from build123d import *

# Parameters (mm, degrees)
UNDERSIDE_COVER_T2_DEPTH         = 2
SKETCH_2_R                       = 1.7
CLOSURE_ONLY_FOUR_M3_HOLES_DEPTH = 2


with BuildPart() as part:
    # 草图1 → Underside_cover_T2 (new body)
    with BuildSketch(Plane.XY):
        with BuildLine():
            Line((41.093704257, -17.903321742), (68.976089412, -17.031997206))
            ThreePointArc((68.976089412, -17.031997206), (69.993731032, -17.065020347), (70.99893626, -17.227030968))
            Line((70.99893626, -17.227030968), (88.335136689, -21.16707652))
            ThreePointArc((88.335136689, -21.16707652), (90.871551504, -20.586309047), (92, -18.241677953))
            Line((92, -18.241677953), (92, 18.241677953))
            ThreePointArc((92, 18.241677953), (90.871551504, 20.586309047), (88.335136689, 21.16707652))
            Line((88.335136689, 21.16707652), (70.99893626, 17.227030968))
            ThreePointArc((70.99893626, 17.227030968), (69.993731032, 17.065020347), (68.976089412, 17.031997206))
            Line((68.976089412, 17.031997206), (41.093704257, 17.903321742))
            ThreePointArc((41.093704257, 17.903321742), (38.912071933, 17.05898058), (38, 14.904785514))
            Line((38, 14.904785514), (38, -14.904785514))
            ThreePointArc((38, -14.904785514), (38.912071933, -17.05898058), (41.093704257, -17.903321742))
        make_face()
    extrude(amount=UNDERSIDE_COVER_T2_DEPTH)

    # 草图2 → Closure_only_four_M3_holes (cut)
    with BuildSketch(Plane.XY.offset(2)):
        with Locations((42, -12)):
            Circle(SKETCH_2_R)
        with Locations((42, 12)):
            Circle(SKETCH_2_R)
        with Locations((75, -13)):
            Circle(SKETCH_2_R)
        with Locations((75, 13)):
            Circle(SKETCH_2_R)
    extrude(amount=-CLOSURE_ONLY_FOUR_M3_HOLES_DEPTH, mode=Mode.SUBTRACT)


solid = part.part
Build history of the part. All positions in model axes, mm. A direction names the side the tool comes from. Coordinates: 2 decimals unless noted, no trailing zeros. Order: outer loops, then holes, each group sorted by start corner. A loop starts at its lowest first (then second) coordinate and runs counter-clockwise, first axis right, second up. Notation, with made-up numbers: (-28.5, 1.25) - (1.5, 1.25) arc R19 ccw to (1.5, 25.25) - close; hole circle Ø11 at (-32.5, 24.5). An arc over 180 degrees is marked (long way). Write item = value, one per line. Start each with the question number.
1) Saw through at D-D on x = 87. Write the cut outline in (y, z).
2) Two-plate mould, pull along X, no slides. Class faces 1 (the face through (92, 0, 1)), 2 (the face through (69.98, -17.064, 0.986)), 3 (the face through (65, 0, 0)): pulls with the +X half, pulls with the -X half, needs draft (parallel to the pull), parting line crosses it, or undercut.
3) Wall check: line 1 along Y through (x, z) = (42, 0.9) (3 decimals); line 2 along X through (y, z) = (-13.5, 1.2); line 3 along Y through (x, z) = (75, 0.75). Give the ranges that are in metal, low to high. Write a range as from..to.
4) Saw through at C-C on y = -12. Write the cut outline in (x, z), then the cut area to 3 significant figures.
5) Saw through at A-A on z = 1. Write the cut outline in (x, y), then the cut area to 3 significant figures.
6) Saw through at B-B on x = 42. Write the cut outline in (y, z) (3 decimals), then the cut area to 3 significant figures.
7) 3-axis set-ups, long thin cutter, end or side, ignore diameter. For faces 4 (the face through (70.008, 17.066, 0.986)), 5 (the face through (79.55, -19.17, 0.99)), 6 (the face through (73.3, -12.93, 1.01)): which of +Z, -Z, +X, -X, +Y, -Y reach the whole face in a straight line?
From the geometry:
q1.outline = (-20.86, 0) - (20.86, 0) - (20.86, 2) - (-20.86, 2) - close
q2.face_1 = pulls with the +X half
q2.face_2 = undercut
q2.face_3 = needs draft
q3.line_1 = -17.875..-13.7, -10.3..10.3, 13.7..17.875
q3.line_2 = 38..41.2, 42.8..73.38, 76.62..92
q3.line_3 = -18.14..-14.7, -11.3..11.3, 14.7..18.14
q4.outline = (38, 0) - (40.3, 0) - (40.3, 2) - (38, 2) - close; (43.7, 0) - (73.63, 0) - (73.63, 2) - (43.7, 2) - close; (76.37, 0) - (92, 0) - (92, 2) - (76.37, 2) - close
q4.area = 95.7 mm^2
q5.outline = (38, -14.9) arc R3 ccw to (41.09, -17.9) - (68.98, -17.03) arc R8 cw to (71, -17.23) - (88.34, -21.17) arc R3 ccw to (92, -18.24) - (92, 18.24) arc R3 ccw to (88.34, 21.17) - (71, 17.23) arc R8 cw to (68.98, 17.03) - (41.09, 17.9) arc R3 ccw to (38, 14.9) - close; hole circle Ø3.4 at (42, -12); hole circle Ø3.4 at (42, 12); hole circle Ø3.4 at (75, -13); hole circle Ø3.4 at (75, 13)
q5.area = 1,930 mm^2
q6.outline = (-17.875, 0) - (-13.7, 0) - (-13.7, 2) - (-17.875, 2) - close; (-10.3, 0) - (10.3, 0) - (10.3, 2) - (-10.3, 2) - close; (13.7, 0) - (17.875, 0) - (17.875, 2) - (13.7, 2) - close
q6.area = 57.9 mm^2
q7.face_4 = +Z, -Z, +Y
q7.face_5 = +Z, -Z, -Y
q7.face_6 = +Z, -Z
